For this review, take the finished solid that the model builds, in its own axes (mm). Face numbers are marked on the shaded views. A direction names the side the tool comes from. Round coordinates to 2 decimals unless told otherwise and drop trailing zeros. Loops run counter-clockwise (first coordinate to the right, second up) from the corner with the lowest first, then second, coordinate; pieces in that order, holes last.
1. Consider section B-B on x = -9. State the section outline as (y, z) points, then the cut area to 3 significant figures.
2. To check wall thickness, follow line 1 along Z through (x, y) = (-4.5, -12); line 2 along Y through (x, z) = (-6.5, 5.5); line 3 along X through (y, z) = (-16, 11). State the ranges of each line that lie inside material, in increasing order.
3. Tool access review of the marked faces 1, 2 and 3: name each direction out of +Z, -Z, +X, -X, +Y, -Y from which nothing blocks a thin tool from reaching the whole face with its end or side.
4. Consider section D-D on z = 3.5. State the section outline as (x, y) points.
5. Clearance check with flat-ended pins moving along their axes: pin 1 Ø8 at (y, z) = (-15, -9.5) entering from +X; pin 2 Ø3 at (x, z) = (-2, 5.5) entering from +Y; pin 3 Ø2 at (x, z) = (-11, -6) entering from -Y; pin 4 Ø20 at (x, z) = (10.5, 1) entering from -Y. State where each tip first meets the part, or that it passes through.
6. Consider section A-A on z = 18. State the section outline as (x, y) points.
7. Consider section C-C on y = -26.5. State the section outline as (x, z) points, then the cut area to 3 significant figures.
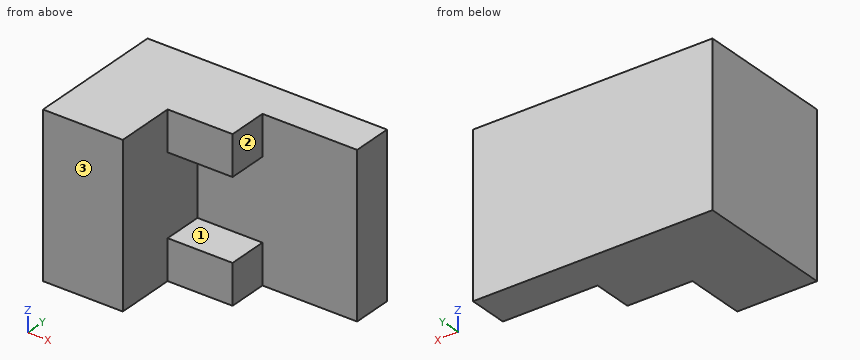
from build123d import *

# Parameters (mm, degrees)
F0_W     = 20
F0_H     = 10
F1_DEPTH = 10
F2_W     = 20
F2_H     = 40
F3_DEPTH = 25
F4_W     = 16.2738668919
F4_H     = 10
F5_DEPTH = 10


with BuildPart() as f1:
    # F0 (on Front) → F1 (new body)
    with BuildSketch(Plane.XZ):
        Polygon((-16.2738668919, 25.1521477103), (-36.2738668919, 25.1521477103), (-36.2738668919, -14.8478522897), (-16.2738668919, -14.8478522897), (-16.2738668919, -4.8478522897), (-16.2738668919, 15.1521477103), align=None)
        with Locations((-6.2738668919, 20.1521477103)):
            Rectangle(F0_W, F0_H)
        Polygon((23.7261331081, 25.1521477103), (3.7261331081, 25.1521477103), (3.7261331081, 15.1521477103), (-16.2738668919, 15.1521477103), (-16.2738668919, -4.8478522897), (3.7261331081, -4.8478522897), (3.7261331081, -14.8478522897), (23.7261331081, -14.8478522897), align=None)
        with Locations((-6.2738668919, -9.8478522897)):
            Rectangle(F0_W, F0_H)
    extrude(amount=F1_DEPTH)

    # F2 (on face) → F3 (join)
    with BuildSketch(Plane.XZ.offset(10)):
        with Locations((-26.2738668919, 5.1521477103)):
            Rectangle(F2_W, F2_H)
    extrude(amount=F3_DEPTH)

    # F4 (on face) → F5 (join)
    with BuildSketch(Plane.XZ.offset(10)):
        with Locations((-8.1369334459, 20.1521477103)):
            Rectangle(F4_W, F4_H)
        with Locations((-8.1369334459, -9.8478522897)):
            Rectangle(F4_W, F4_H)
    extrude(amount=F5_DEPTH)


solid = f1.part
Resolved:
1. outline: (-20, -14.85) - (0, -14.85) - (0, 25.15) - (-20, 25.15) - (-20, 15.15) - (-10, 15.15) - (-10, -4.85) - (-20, -4.85) - close
1. area: 600 mm2
2. line 1: z = -14.85 to -4.85, 15.15 to 25.15
2. line 2: y = -10 to 0
2. line 3: x = -36.27 to -16.27
3. face 1: +X, -Y
3. face 2: +Z, -Z, +X, -Y
3. face 3: +Z, -Z, +X, -X, -Y
4. outline: (-36.27, -35) - (-16.27, -35) - (-16.27, -10) - (23.73, -10) - (23.73, 0) - (-36.27, 0) - close
5. pin 1: stops at x = 0
5. pin 2: stops at y = 0
5. pin 3: stops at y = -20
5. pin 4: stops at y = -10
6. outline: (-36.27, -35) - (-16.27, -35) - (-16.27, -20) - (0, -20) - (0, -10) - (23.73, -10) - (23.73, 0) - (-36.27, 0) - close
7. outline: (-36.27, -14.85) - (-16.27, -14.85) - (-16.27, 25.15) - (-36.27, 25.15) - close
7. area: 800 mm2
